Check sheet for the modelled part. Datum: model origin and axes. Units: mm. A direction names the side the tool comes from. Round coordinates to 2 decimals unless told otherwise and drop trailing zeros. Loops run counter-clockwise (first coordinate to the right, second up) from the corner with the lowest first, then second, coordinate; pieces in that order, holes last. Notation, with made-up numbers: (81, 87) - (88, 87) arc R30 cw to (88, 110) - close; hole circle Ø7 at (-14.5, 9). An arc over 180 degrees is marked (long way). Answer in a Markdown table with one row per item. Add a question column.
(1) Cross-section at B-B on z = 3. Enter the section's corners in (x, y).
(2) Gauge pin test, flat end, axial feed: pin 1 (1.5 mm diameter, centred on y = -110.5, z = 3, fed in from -X). Record the tip position at first contact, or that the pin passes through.
(3) Cross-section at C-C on x = 31. Enter the section's corners in (y, z).
(4) Thickness scan on line 1 along Y through (x, z) = (31.25, 3); line 2 along Y through (x, z) = (28.25, 3.3); line 3 along Y through (x, z) = (28.75, 2.35). Record the ranges inside material, lowest first.
(5) Mould release check, pull along Y, two halves, no side actions. Record for faces 3 (the cylindrical face through (30.295, -109.184, 2.805)), 4 (the flat face through (25.365, -84, 3)), 5 (the cylindrical face through (45.902, -74.828, 2.958)), 6 (the flat face through (38, -50.671, 3)): +Y half, -Y half, draft (parallel to the pull), parting line (faces both ways), or undercut.
(6) Access from +Z, -Z, +X, -X, +Y, -Y to the whole of each face (thin tool, end or side, straight path). Record for faces 1 (the flat face through (50.365, -84, 3)), 2 (the cylindrical face through (30.295, -57.135, 2.675)).
(7) Cross-section at A-A on y = -77.5. Enter the section's corners in (x, z), then the cut area to 3 significant figures.
from build123d import *

# Parameters (mm, degrees)
ESQUISSE1_W             = 25
ESQUISSE1_H             = 65
ESQUISSE1_R             = 1
ESQUISSE1_R_2           = 4
BOSS_EXTRU_1_DEPTH      = 6
ESQUISSE4_R             = 1.5
ENL_V_MAT_EXTRU_3_DEPTH = 10


with BuildPart() as part:
    # Esquisse1 → Boss.-Extru.1 (new body)
    with BuildSketch(Plane.XY):
        with Locations((37.864568032, -83.170745263)):
            Rectangle(ESQUISSE1_W, ESQUISSE1_H)
        with Locations((29.364568032, -75.670745263)):
            Circle(ESQUISSE1_R, mode=Mode.SUBTRACT)
        with Locations((37.364568032, -67.670745263)):
            Circle(ESQUISSE1_R, mode=Mode.SUBTRACT)
        with Locations((45.364568032, -75.670745263)):
            Circle(ESQUISSE1_R, mode=Mode.SUBTRACT)
        with Locations((37.364568032, -83.670745263)):
            Circle(ESQUISSE1_R, mode=Mode.SUBTRACT)
        with Locations((37.364568032, -75.670745263)):
            Circle(ESQUISSE1_R_2, mode=Mode.SUBTRACT)
    extrude(amount=BOSS_EXTRU_1_DEPTH)

    # Esquisse4 → Enlèv. mat.-Extru.3 (cut)
    with BuildSketch(Plane.ZY.offset(-25.364568032)):
        with Locations((3, -55.670745263)):
            Circle(ESQUISSE4_R)
        with Locations((3, -110.670745263)):
            Circle(ESQUISSE4_R)
    extrude(amount=-ENL_V_MAT_EXTRU_3_DEPTH, mode=Mode.SUBTRACT)


solid = part.part
Answers:
| question | item | result |
|---|---|---|
| 1 | outline | (25.36, -115.67) - (50.36, -115.67) - (50.36, -50.67) - (25.36, -50.67) - (25.36, -54.17) - (35.36, -54.17) - (35.36, -57.17) - (25.36, -57.17) - (25.36, -109.17) - (35.36, -109.17) - (35.36, -112.17) - (25.36, -112.17) - close; hole circle Ø2 at (29.36, -75.67); hole circle Ø8 at (37.36, -75.67); hole circle Ø2 at (37.36, -83.67); hole circle Ø2 at (37.36, -67.67); hole circle Ø2 at (45.36, -75.67) |
| 2 | pin 1 | stops at x = 35.36 |
| 3 | outline | (-115.67, 0) - (-50.67, 0) - (-50.67, 6) - (-115.67, 6) - close; hole circle Ø3 at (-110.67, 3); hole circle Ø3 at (-55.67, 3) |
| 4 | line 1 | y = -115.67 to -112.17, -109.17 to -57.17, -54.17 to -50.67 |
| 4 | line 2 | y = -115.67 to -112.14, -109.2 to -57.14, -54.2 to -50.67 |
| 4 | line 3 | y = -115.67 to -112.02, -109.32 to -76.46, -74.88 to -57.02, -54.32 to -50.67 |
| 5 | face 3 | undercut |
| 5 | face 4 | draft |
| 5 | face 5 | undercut |
| 5 | face 6 | +Y half |
| 6 | face 1 | +Z, -Z, +X, +Y, -Y |
| 6 | face 2 | -X |
| 7 | outline | (25.36, 0) - (33.81, 0) - (33.81, 6) - (25.36, 6) - close; (40.92, 0) - (50.36, 0) - (50.36, 6) - (40.92, 6) - close |
| 7 | area | 107 mm^2 |
